Design review of the part shown in the three views and the two pictorial views. Dimensions are in mm from the part's minimum x, y and z. Give positions to 0.01 mm unless a question says otherwise; leave off trailing zeros. Order: outer loops, then holes, each group sorted by start corner. A loop starts at its lowest first (then second) coordinate and runs counter-clockwise, first axis right, second up.
Item 1: For P1, Ø1.5, axis at x = 7.5, y = 4.5, coming from the +Z side, flat-tipped, find the tip position at first contact; note if it passes through.
Item 2: Consider section B-B (x = 5). Give the boundary of the cut face in (y, z), plus the area to 3 significant figures.
Item 3: Consider section A-A (y = 5). Give the boundary of the cut face in (x, z), plus the area to 3 significant figures.
Item 4: For probe 1 along X at (y, z) = (5, 3.15); probe 2 along Y at (x, z) = (5, 1.3); probe 3 along X at (y, z) = (5.5, 0.35), list the stretches that pass through material, from the lowest coordinate up.
Item 5: Consider section C-C (z = 2.2). Give the boundary of the cut face in (x, y), plus the area to 3 significant figures.
Item 6: The part is to be moulded in two halves that separate along Y. For the marked faces 1, 2 and 3, say which applies: released by +Y, released by -Y, zero draft, split by the parting line, or undercut.
Item 7: Consider section D-D (z = 1.05). Give the boundary of the cut face in (x, y).
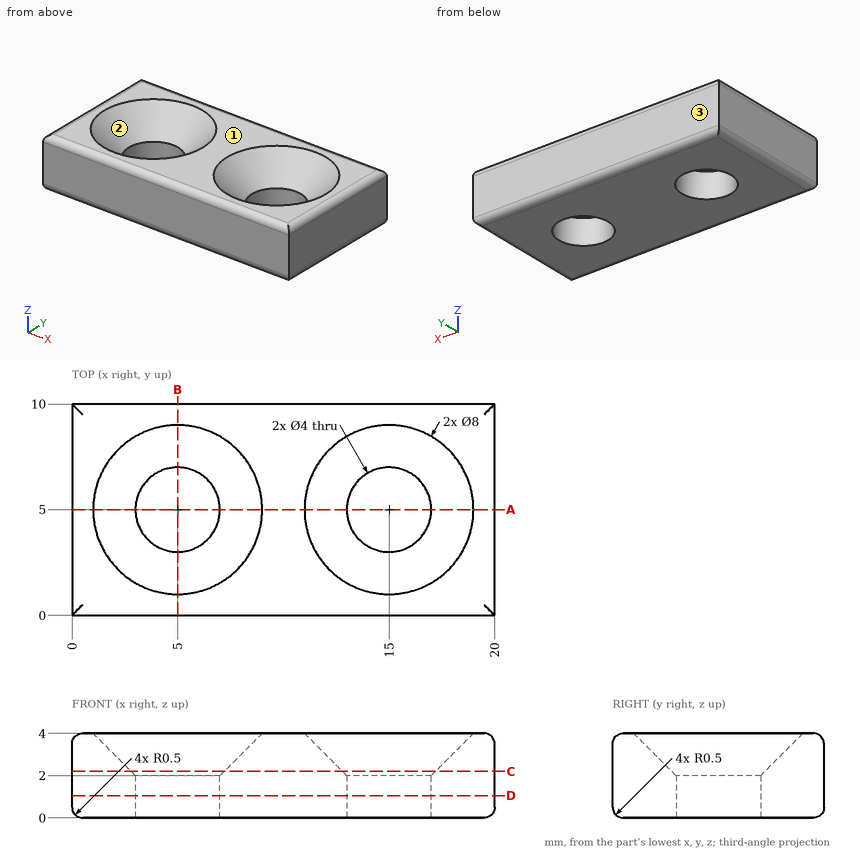
Resolved:
1. P1: stops at z = 3.3
2. outline: (0, 0.5) arc R0.5 ccw to (0.5, 0) - (3, 0) - (3, 2) - (1, 4) - (0.5, 4) arc R0.5 ccw to (0, 3.5) - close; (7, 0) - (9.5, 0) arc R0.5 ccw to (10, 0.5) - (10, 3.5) arc R0.5 ccw to (9.5, 4) - (9, 4) - (7, 2) - close
2. area: 19.8 mm2
3. outline: (0, 0.5) arc R0.5 ccw to (0.5, 0) - (3, 0) - (3, 2) - (1, 4) - (0.5, 4) arc R0.5 ccw to (0, 3.5) - close; (7, 0) - (13, 0) - (13, 2) - (11, 4) - (9, 4) - (7, 2) - close; (17, 0) - (19.5, 0) arc R0.5 ccw to (20, 0.5) - (20, 3.5) arc R0.5 ccw to (19.5, 4) - (19, 4) - (17, 2) - close
3. area: 39.8 mm2
4. probe 1: x = 0 to 1.85, 8.15 to 11.85, 18.15 to 20
4. probe 2: y = 0 to 3, 7 to 10
4. probe 3: x = 0.02 to 3.06, 6.94 to 13.06, 16.94 to 19.98
5. outline: (0, 0) - (20, 0) - (20, 10) - (0, 10) - close; hole circle Ø4.4 at (5, 5); hole circle Ø4.4 at (15, 5)
5. area: 170 mm2
6. face 1: zero draft
6. face 2: undercut
6. face 3: released by +Y
7. outline: (0, 0) - (20, 0) - (20, 10) - (0, 10) - close; hole circle Ø4 at (5, 5); hole circle Ø4 at (15, 5)
